Design review of the part shown in the three views and the two pictorial views. Dimensions are in mm from the part's minimum x, y and z. A direction names the side the tool comes from. Give positions to 0.01 mm unless a question says otherwise; leave off trailing zeros. Loops run counter-clockwise (first coordinate to the right, second up) from the corner with the lowest first, then second, coordinate; pieces in that order, holes last. Notation, with made-up numbers: (62.5, 86.25) -> (115.5, 86.25) arc R26 ccw to (115.5, 125.25) -> close; hole circle Ø11 at (38, 23.25). An arc over 180 degrees is marked (long way). Answer as CSV lines item,"result". Start each with the question number.
Item 1: The part is to be moulded in two halves that separate along Z. For the marked faces 3, 4 and 5, say which applies: +Z half, -Z half, draft (parallel to the pull), parting line (faces both ways), or undercut.
Item 2: For L1, parallel to Z at x = 66.5, y = 3.9; L2, parallel to Z at x = 66.5, y = 1.8; L3, parallel to X at y = 3.2, z = 53.5, list the stretches that pass through material, from the lowest coordinate up. Write a range as from..to.
Item 3: Add section B-B on y = 10.5. State the section outline as (x, z) points.
Item 4: Clearance check with flat-ended pins moving along their axes: P1, Ø5, axis at x = 24, z = 35.5, coming from the +Y side; P2, Ø2.5, axis at x = 1, z = 41.5, coming from the +Y side; P3, Ø5, axis at x = 6.5, z = 56, coming from the +Y side. State where each tip first meets the part, or that it passes through.
Item 5: Add section A-A on x = 5. State the section outline as (y, z) points.
Item 6: Add section C-C on z = 6. State the section outline as (x, y) points.
Item 7: Add section D-D on z = 36.5. State the section outline as (x, y) points, plus the area to 3 significant figures.
Item 8: Machinability: for the marked faces 1 and 2, which of the approach directions +Z, -Z, +X, -X, +Y, -Y give a long, thin tool a straight path to every point of the face, cutting with its end or side? Answer none if there is none.
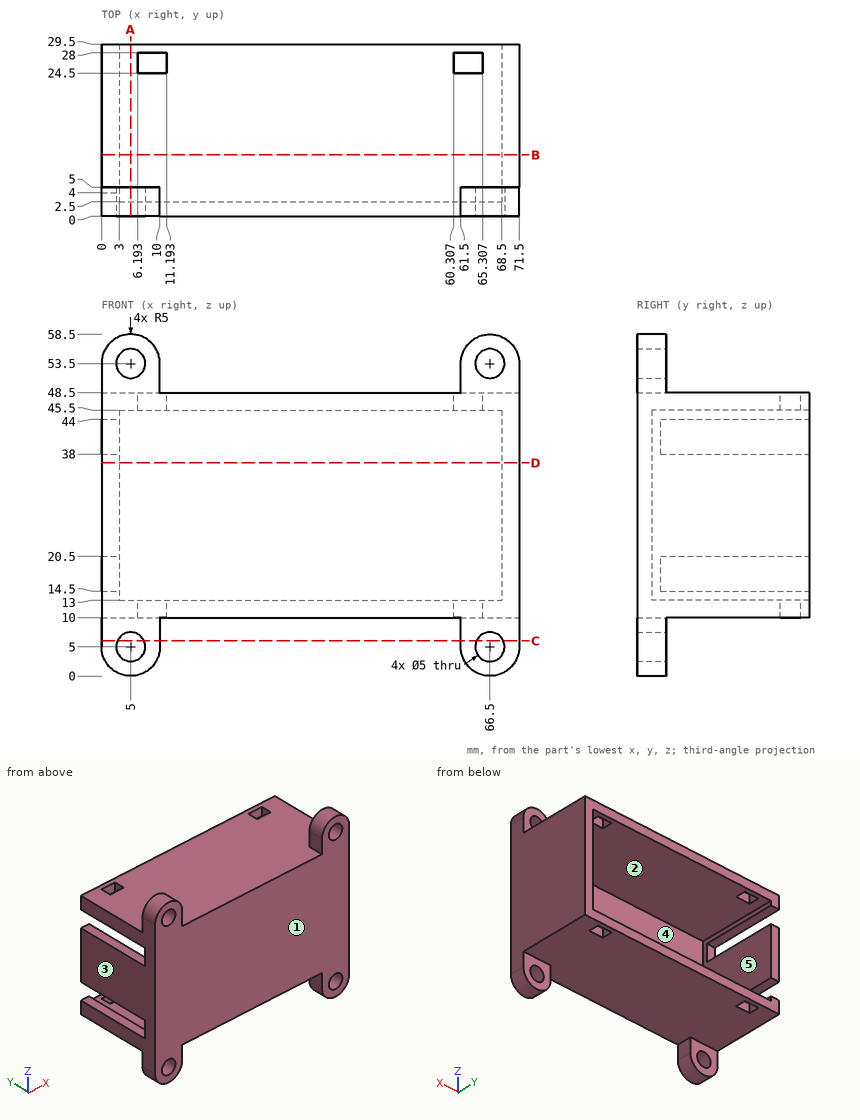
Computed values:
1,face 3,"draft"
1,face 4,"undercut"
1,face 5,"undercut"
2,L1,"0..2.5, 7.5..13, 45.5..51, 56..58.5"
2,L2,"0..2.5, 7.5..51, 56..58.5"
2,L3,"0..2.5, 7.5..10, 61.5..64, 69..71.5"
3,outline,"(0, 10) -> (71.5, 10) -> (71.5, 48.5) -> (0, 48.5) -> (0, 44) -> (3, 44) -> (3, 45.5) -> (68.5, 45.5) -> (68.5, 13) -> (3, 13) -> (3, 14.5) -> (0, 14.5) -> close; (0, 20.5) -> (3, 20.5) -> (3, 38) -> (0, 38) -> close"
4,P1,"y = 2.5"
4,P2,"y = 4"
4,P3,"y = 5"
5,outline,"(0, 0) -> (5, 0) -> (5, 2.5) -> (0, 2.5) -> close; (0, 7.5) -> (5, 7.5) -> (5, 10) -> (29.5, 10) -> (29.5, 13) -> (2.5, 13) -> (2.5, 45.5) -> (29.5, 45.5) -> (29.5, 48.5) -> (5, 48.5) -> (5, 51) -> (0, 51) -> close; (0, 56) -> (5, 56) -> (5, 58.5) -> (0, 58.5) -> close"
6,outline,"(0, 0) -> (2.71, 0) -> (2.71, 5) -> (0, 5) -> close; (7.29, 0) -> (10, 0) -> (10, 5) -> (7.29, 5) -> close; (61.5, 0) -> (64.21, 0) -> (64.21, 5) -> (61.5, 5) -> close; (68.79, 0) -> (71.5, 0) -> (71.5, 5) -> (68.79, 5) -> close"
7,outline,"(0, 0) -> (71.5, 0) -> (71.5, 29.5) -> (68.5, 29.5) -> (68.5, 2.5) -> (3, 2.5) -> (3, 29.5) -> (0, 29.5) -> close"
7,area,"341 mm²"
8,face 1,"+Z, -Z, +X, -X, -Y"
8,face 2,"+Y"
